Autodesk Inventor part; units mm, degrees
ref_plane "YZ Plane" through (0, 0, 0) normal (1, 0, 0) x (0, 1, 0)
ref_plane "XZ Plane" through (0, 0, 0) normal (0, 1, 0) x (-1, 0, 0)
ref_plane "XY Plane" through (0, 0, 0) normal (0, 0, 1) x (1, 0, 0)
sketch "Sketch1" plane through (0, 0, 0) normal (0, 1, 0) x (-1, 0, 0)
  circle A0 centre (0, 0) radius 25 construction
  line L0 (44.45, 0) -> (-44.45, 0) construction
  line L1 (0, -44.45) -> (0, 44.45) construction
  circle A1 centre (0, 0) radius 31.75
  circle A2 centre (0, 0) radius 16 construction
  line L2 (11.3137, 11.3137) -> (-11.3137, -11.3137) construction
  line L3 (-11.3137, 11.3137) -> (11.3137, -11.3137) construction
  line L4 (-20, 20) -> (20, 20) construction
  line L5 (20, 20) -> (20, -20) construction
  line L6 (20, -20) -> (-20, -20) construction
  line L7 (-20, -20) -> (-20, 20) construction
  line L8 (-20, 20) -> (20, -20) construction
  line L9 (20, 20) -> (-20, -20) construction
  line L10 (16, -20) -> (16, -27.4238)
  line L11 (16, -20) -> (-24.6589, -20)
  line L12 (20, -16) -> (27.4238, -16)
  line L13 (20, -16) -> (20, 24.6589)
  line L14 (16, -16) -> (-16, -16)
  line L15 (-16, -16) -> (-16, 16)
  line L16 (-16, 16) -> (16, 16)
  line L17 (16, 16) -> (16, -16)
  point P0 (0, 25)
  point P1 (25, 0)
  point P2 (0, -25)
  point P3 (-25, 0)
  point P4 (-16, 16)
  dimension "M6ClearancePatternDiameter" = 50
  dimension "diameter" = 63.5
  dimension "M3TappedPatternEdge" = 32
  dimension "d3" = 45
  dimension "d20" = 40
  dimension "d21" = 40
extrude "Extrusion1" add sketch "Sketch1" against normal blind 12 contours A1 L12 L13 | L13 L12 A1 L10 L11 | L11 L10 A1 | L14 L15 L16 L17
extrude "Extrusion3" add sketch "Sketch1" along normal blind 1 contours A1 L12 L13 | L11 L10 A1
hole "M3Tapped" at (-16, 0, -16) at (16, 0, -16) at (16, 0, 16) at (-16, 0, 16) direction (0, -1, 0) diameter 2.459 depth 8.8 tip angle 118
hole "Hole4" at (0, 0, 25) at (-25, 0, 0) at (0, 0, -25) at (25, 0, 0) direction (0, -1, 0) diameter 6.4 end through all counterbore diameter 11 counterbore depth 6.8
sketch "Sketch2" plane through (0, 0, 0) normal (0, -1, 0) x (1, 0, 0)
  circle A0 centre (25, 0) radius 5.5
  arc A1 (2.2913, -20) -> (-2.2913, -20) centre (0, -25) ccw
  arc A2 (-2.2913, -20) -> (2.2913, -20) centre (0, -25) ccw
  circle A3 centre (0, 25) radius 5.5
  line L0 (-20, 24.6589) -> (-20, 2.2913)
  line L1 (-20, 2.2913) -> (-20, -2.2913)
  line L2 (-20, -2.2913) -> (-20, -16)
  line L3 (-20, -16) -> (-27.4238, -16)
  line L4 (-16, -27.4238) -> (-16, -20)
  line L5 (-16, -20) -> (-2.2913, -20)
  line L6 (-2.2913, -20) -> (2.2913, -20)
  line L7 (2.2913, -20) -> (24.6589, -20)
  arc A4 (-20, -2.2913) -> (-20, 2.2913) centre (-25, 0) ccw
  arc A5 (-20, 2.2913) -> (-20, -2.2913) centre (-25, 0) ccw
  arc A6 (-27.4238, -16) -> (-16, -27.4238) centre (0, 0) ccw
  arc A7 (-16, -27.4238) -> (24.6589, -20) centre (0, 0) ccw
  arc A8 (-20, 24.6589) -> (-27.4238, -16) centre (0, 0) ccw
  arc A9 (24.6589, -20) -> (-20, 24.6589) centre (0, 0) ccw
  circle A10 centre (16, 16) radius 1.2295
  circle A11 centre (-16, -16) radius 1.2295
  circle A12 centre (16, -16) radius 1.2295
  circle A13 centre (-16, 16) radius 1.2295
extrude "Extrusion4" cut sketch "Sketch2" against normal through all contours A2 L6 | L1 A5
equation "\"d21\" = d20"
equation "\"d4\" = thickness"
equation "\"d24\" = recessDepth"
equation "\"d40\" = recessDepth"
equation "\"thickness\" = 12"
equation "\"recessDepth\" = 1"
properties part number "FAB-OX0005"
Model file for the job. Use its own axes, mm. A direction names the side the tool comes from. Give positions to 0.01 mm unless a question says otherwise; leave off trailing zeros. Write each loop counter-clockwise with the first axis right and the second up, starting at its lowest first coordinate (ties: lowest second). Pieces come first, ordered by that corner, then holes. Notation, with made-up numbers: (80, 7.25) - (117, 7.25) arc R21 ccw to (117, 28.25) - close; hole circle Ø11 at (-5.5, 26). An arc over 180 degrees is marked (long way). One line per question, with ' | ' between items. Start each with the question number.
(1) Slice it at A-A on x = 0. Write the cut outline in (y, z), plus the area to 3 significant figures.
(2) 3-axis set-ups, long thin cutter, end or side, ignore diameter. For faces 1 (the face through (15.631, -4.462, 17.173)), 2 (the face through (-0.1, -9.4, -28.2)): which of +Z, -Z, +X, -X, +Y, -Y reach the whole face in a straight line?
(3) Two-plate mould, pull along Z, no slides. Class faces 3 (the face through (19.547, -3.448, -0.716)), 4 (the face through (0, -12, 0)), 5 (the face through (-30.03, -5.59, -10.31)): +Z half, -Z half, draft (parallel to the pull), parting line (faces both ways), or undercut.
(4) Wall check: line 1 along Z through (x, y) = (0, -9.55); line 2 along X through (y, z) = (-2.75, 0); line 3 along Z through (x, y) = (-16, -6). Give the ranges that are in metal, low to high. Write a range as from..to.
(5) Slice it at C-C on y = -5.75. Give the number of separate pieces and of enclosed holes in the cut face, plus the area to 3 significant figures.
(6) Slice it at B-B on z = 0. Write the cut outline in (x, y), plus the area to 3 significant figures.
(7) Pin check, flat tips, straight feed: P1, Ø12, axis at x = -1.5, z = 22.5, coming from the +Y side; P2, Ø1.5, axis at x = 19, y = -4, coming from the +Z side; P3, Ø10, axis at x = 0, z = -25, coming from the +Y side. Stop position of each tip, or through.
(8) Slice it at D-D on z = -23. Write the cut outline in (x, y), plus the area to 3 significant figures.
Results below:
1) outline: (-12, -31.75) - (1, -31.75) - (1, -30.5) - (-6.8, -30.5) - (-6.8, -28.2) - (-12, -28.2) - close; (-12, -21.8) - (-6.8, -21.8) - (-6.8, -19.5) - (0, -19.5) - (0, 19.5) - (-6.8, 19.5) - (-6.8, 21.8) - (-12, 21.8) - close; (-12, 28.2) - (-6.8, 28.2) - (-6.8, 30.5) - (0, 30.5) - (0, 31.75) - (-12, 31.75) - close | area: 547 mm^2
2) face 1: +Y | face 2: +Y, -Y
3) face 3: undercut | face 4: draft | face 5: parting line
4) line 1: -31.75..-28.2, -21.8..21.8, 28.2..31.75 | line 2: -31.75..-30.5, -19.5..19.5, 30.5..31.75 | line 3: -27.42..-17.23, -14.77..14.77, 17.23..27.42
5) separate pieces: 1 | enclosed holes: 8 | area: 2,770 mm^2
6) outline: (-31.75, -12) - (-28.2, -12) - (-28.2, -6.8) - (-30.5, -6.8) - (-30.5, 1) - (-31.75, 1) - close; (-21.8, -12) - (21.8, -12) - (21.8, -6.8) - (19.5, -6.8) - (19.5, 0) - (-19.5, 0) - (-19.5, -6.8) - (-21.8, -6.8) - close; (28.2, -12) - (31.75, -12) - (31.75, 0) - (30.5, 0) - (30.5, -6.8) - (28.2, -6.8) - close | area: 547 mm^2
7) P1: y = 0 | P2: z = 25.98 | P3: y = -6.8
8) outline: (-21.89, -12) - (-2.5, -12) - (-2.5, -6.8) - (-5.12, -6.8) - (-5.12, 1) - (-16, 1) - (-16, 0) - (-21.89, 0) - close; (2.5, -12) - (21.89, -12) - (21.89, 1) - (5.12, 1) - (5.12, -6.8) - (2.5, -6.8) - close | area: 457 mm^2
